Geometry check sheet. Reference: the model listing, model coordinates, mm. Face numbers are marked on the shaded views. A direction names the side the tool comes from. Round coordinates to 2 decimals unless told otherwise and drop trailing zeros. Loops run counter-clockwise (first coordinate to the right, second up) from the corner with the lowest first, then second, coordinate; pieces in that order, holes last. Notation, with made-up numbers: M 87,57.25 L 95,57.25 A30 cw 95,85.25 Z; hole C 11,66 d1. An arc over 180 degrees is marked long. Use one line per item in the form item = value. Start each with the question number.
1. Cross-section at A-A (x = 0). Record the boundary of the cut face in (y, z), then the cut area to 3 significant figures.
2. Cross-section at C-C (y = 7). Record the boundary of the cut face in (x, z), then the cut area to 3 significant figures.
3. Cross-section at B-B (z = 0). Record the boundary of the cut face in (x, y), then the cut area to 3 significant figures.
4. Set-up check for the marked faces 1, 2, 3 and 4: record each of +Z, -Z, +X, -X, +Y, -Y from which the full face is reachable in a straight line by a thin tool's end or side.
5. Draft check along X on the marked faces 5, 6, 7 and 8. Enter one of: pulls with the +X half, pulls with the -X half, needs draft (parallel to the pull), parting line crosses it, or undercut.
6. Cross-section at D-D (z = 35). Record the boundary of the cut face in (x, y).
7. Material ranges on line 1 (X direction, y = 0.7, z = 35); line 2 (X direction, y = 14, z = 0); line 3 (Y direction, x = 21, z = -1.5), recorded low to high.
8. Go/stop test with flat-tipped pins: pin 1 (5 mm diameter, centred on y = 10.5, z = 32.5, fed in from +X); pin 2 (2 mm diameter, centred on x = 0, z = 35, fed in from -Y); pin 3 (9 mm diameter, centred on x = 0, z = 39.5, fed in from +Y); pin 4 (1 mm diameter, centred on y = 11, z = -31.5, fed in from -X). Record where each tip stops, or that it passes through.
```python
from build123d import *

# Parameters (mm, degrees)
EXTRUDE_2_DEPTH      = 1
SKETCH_6_R           = 27.5
SKETCH_6_R_2         = 26.5
EXTRUDE_3_DEPTH      = 17
EXTRUDE_4_REACH      = 97.814
EXTRUDE_4_END_RADIUS = 27.5
SKETCH_8_W           = 1
SKETCH_8_H           = 17
CUT_EXTRUDE_2_DEPTH  = 20
SKETCH_11_R          = 1.65
CUT_EXTRUDE_3_DEPTH  = 20


with BuildPart() as part:
    # 草图3 → 凸台-拉伸2 (new body)
    with BuildSketch(Plane(origin=(0, 0, 0), x_dir=(1, 0, 0), z_dir=(0, 1, 0))):
        with BuildLine():
            Line((-10, 25.617376915), (-10, 45))
            Line((-10, 45), (10, 45))
            Line((10, 45), (10, 25.617376915))
            ThreePointArc((10, 25.617376915), (27.5, 0), (10, -25.617376915))
            Line((10, -25.617376915), (10, -45))
            Line((10, -45), (-10, -45))
            Line((-10, -45), (-10, -25.617376915))
            ThreePointArc((-10, -25.617376915), (-27.5, 0), (-10, 25.617376915))
        make_face()
    extrude(amount=EXTRUDE_2_DEPTH)

    # 草图6 → 凸台-拉伸3 (add)
    with BuildSketch(Plane(origin=(0, 1, 0), x_dir=(1, 0, 0), z_dir=(0, 1, 0))):
        with Locations(Location((0, 0, 0), (0, 0, 68.676313737))):
            Circle(SKETCH_6_R)
        with Locations(Location((0, 0, 0), (0, 0, 270))):
            Circle(SKETCH_6_R_2, mode=Mode.SUBTRACT)
    extrude(amount=EXTRUDE_3_DEPTH)

    # 凸台-拉伸4: up to this cylinder (the profile starts outside it)
    extrude_4_end = Plane(origin=(0, 9.5, 0), z_dir=(0, -1, 0)) * Cylinder(EXTRUDE_4_END_RADIUS, 251.628, mode=Mode.PRIVATE)
    # 草图8 → 凸台-拉伸4 (add, up to the surface)
    with BuildSketch(Plane.XY.offset(45), mode=Mode.PRIVATE) as extrude_4_sk1:
        with Locations((-9.5, 9.5)):
            Rectangle(SKETCH_8_W, SKETCH_8_H)
    extrude_4_tool1 = extrude(extrude_4_sk1.sketch, amount=-EXTRUDE_4_REACH, mode=Mode.PRIVATE) - extrude_4_end
    # 草图8 → 凸台-拉伸4 (add, up to the surface)
    with BuildSketch(Plane.XY.offset(45), mode=Mode.PRIVATE) as extrude_4_sk2:
        with Locations((9.5, 9.5)):
            Rectangle(SKETCH_8_W, SKETCH_8_H)
    extrude_4_tool2 = extrude(extrude_4_sk2.sketch, amount=-EXTRUDE_4_REACH, mode=Mode.PRIVATE) - extrude_4_end
    extrude_4 = extrude_4_tool1.solids().sort_by_distance((-9.5, 9.5, 45))[0] + extrude_4_tool2.solids().sort_by_distance((9.5, 9.5, 45))[0]
    add(extrude_4)

    # 草图9 → 切除-拉伸2 (cut)
    with BuildSketch(Plane.ZY.offset(10)):
        Polygon((28.117376915, 18), (45, 2), (45, 18), align=None)
    cut_extrude_2 = extrude(amount=-CUT_EXTRUDE_2_DEPTH, mode=Mode.SUBTRACT)

    # 镜向1: 凸台-拉伸4, 切除-拉伸2 across plane
    add(extrude_4.mirror(Plane.XY))
    add(cut_extrude_2.mirror(Plane.XY), mode=Mode.SUBTRACT)

    # 草图11 → 切除-拉伸3 (cut)
    with BuildSketch(Plane(origin=(0, 1, 0), x_dir=(1, 0, 0), z_dir=(0, 1, 0))):
        with Locations(Location((0, 35, 0), (0, 0, 270))):
            Circle(SKETCH_11_R)
        with Locations(Location((0, -35, 0), (0, 0, 270))):
            Circle(SKETCH_11_R)
    extrude(amount=-CUT_EXTRUDE_3_DEPTH, mode=Mode.SUBTRACT)


solid = part.part
```
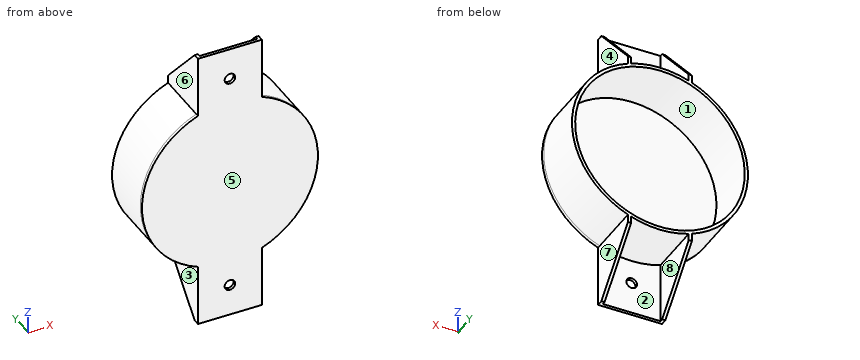
Reported:
q1.outline = M 0,-45 L 1,-45 L 1,-36.65 L 0,-36.65 Z; M 0,-33.35 L 1,-33.35 L 1,-27.5 L 18,-27.5 L 18,-26.5 L 1,-26.5 L 1,26.5 L 18,26.5 L 18,27.5 L 1,27.5 L 1,33.35 L 0,33.35 Z; M 0,36.65 L 1,36.65 L 1,45 L 0,45 Z
q1.area = 117 mm²
q2.outline = M -10,-39.72 L -9,-39.72 L -9,-25.99 A27.5 ccw 9,-25.99 L 9,-39.72 L 10,-39.72 L 10,-25.62 A27.5 ccw 10,25.62 L 10,39.72 L 9,39.72 L 9,25.99 A27.5 ccw -9,25.99 L -9,39.72 L -10,39.72 L -10,25.62 A27.5 ccw -10,-25.62 Z; hole C 0,0 d53
q2.area = 225 mm²
q3.outline = M -27.5,0 L 27.5,0 L 27.5,18 L 26.5,18 L 26.5,1 L -26.5,1 L -26.5,18 L -27.5,18 Z
q3.area = 89.0 mm²
q4.face_1 = +Y
q4.face_2 = -Z, +Y
q4.face_3 = -Z, -X, +Y, -Y
q4.face_4 = +Z, +X, +Y, -Y
q5.face_5 = needs draft
q5.face_6 = pulls with the -X half
q5.face_7 = pulls with the +X half
q5.face_8 = undercut
q6.outline = M -10,0 L -1.65,0 L -1.65,1 L -9,1 L -9,11.48 L -10,11.48 Z; M 1.65,0 L 10,0 L 10,11.48 L 9,11.48 L 9,1 L 1.65,1 Z
q7.line_1 = -10 to -1.65, 1.65 to 10
q7.line_2 = -27.5 to -26.5, 26.5 to 27.5
q7.line_3 = 0 to 1
q8.pin_1 = 10
q8.pin_2 = through
q8.pin_3 = 1
q8.pin_4 = -10
